Could you check a few things on this model? Use its own coordinates, in mm. Round coordinates to 2 decimals unless told otherwise and drop trailing zeros. Write each loop counter-clockwise with the first axis right and the second up, starting at its lowest first coordinate (ties: lowest second). Pieces come first, ordered by that corner, then holes. Notation, with made-up numbers: (70, 81) -> (109, 81) arc R19 ccw to (109, 111) -> close; hole circle Ø2 at (82, 26). An arc over 180 degrees is marked (long way). Answer in a Markdown table with one row per item.
from build123d import *

# Parameters (mm, degrees)
F4_R = 0.9


with BuildPart() as f1:
    # F0 (on Front) → F1 (revolve)
    with BuildSketch(Plane.XZ):
        Polygon((-70.710678, 0), (0, 0), (0, 70.710678), align=None)
    revolve(axis=Axis((0, 0, 35.355339), (0, 0, 1)))

    # F2 (on Front) → F3 (revolve, cut)
    with BuildSketch(Plane.XZ):
        with BuildLine():
            ThreePointArc((-47, 0), (0, -47), (47, 0))
            Line((47, 0), (-47, 0))
        make_face()
    revolve(axis=Axis((0, 0, 0), (1, 0, 0)), mode=Mode.SUBTRACT)

    # F4
    f4_edges = [f1.edges().sort_by_distance(p)[0] for p in [
        (70.710678, 0, 0),
    ]]
    fillet(f4_edges, radius=F4_R)


solid = f1.part
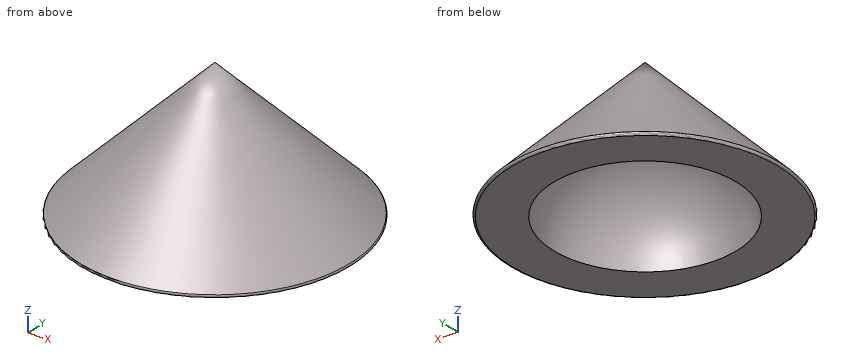
1) For pin 1 (1.5 mm diameter, centred on x = -22.5, y = 32.5, fed in from +Z); pin 2 (12 mm diameter, centred on y = -6.5, z = 33.5, fed in from -X); pin 3 (3 mm diameter, centred on x = 55, y = 24, fed in from +Z); pin 4 (8 mm diameter, centred on x = -51.5, y = 21, fed in from -Z), each with a flat end and sliding along its axis, tell me the tip position at first contact or that it passes through.
Findings:
| item | result |
|---|---|
| pin 1 | stops at z = 31.93 |
| pin 2 | stops at x = -42.78 |
| pin 3 | stops at z = 12.2 |
| pin 4 | stops at z = 0 |
2) Please list where these lines run through material, in increasing order: line 1 (Y direction, x = 25, z = 16); line 2 (Y direction, x = -2, z = 28); line 3 (X direction, y = 12.5, z = 14).
Findings:
| item | result |
|---|---|
| line 1 | y = -48.66 to -36.44, 36.44 to 48.66 |
| line 2 | y = -42.66 to -37.7, 37.7 to 42.66 |
| line 3 | x = -55.32 to -43.09, 43.09 to 55.32 |
3) Imagine slicing it at A-A, the plane z = 15. Please give me the cut outline in (x, y).
Findings:
| item | result |
|---|---|
| outline | circle Ø111.42 at (0, 0); hole circle Ø89.08 at (0, 0) |
4) Imagine slicing it at B-B, the plane z = 49. Please give me the cut outline in (x, y), plus the area to 3 significant figures.
Findings:
| item | result |
|---|---|
| outline | circle Ø43.42 at (0, 0) |
| area | 1,480 mm^2 |
